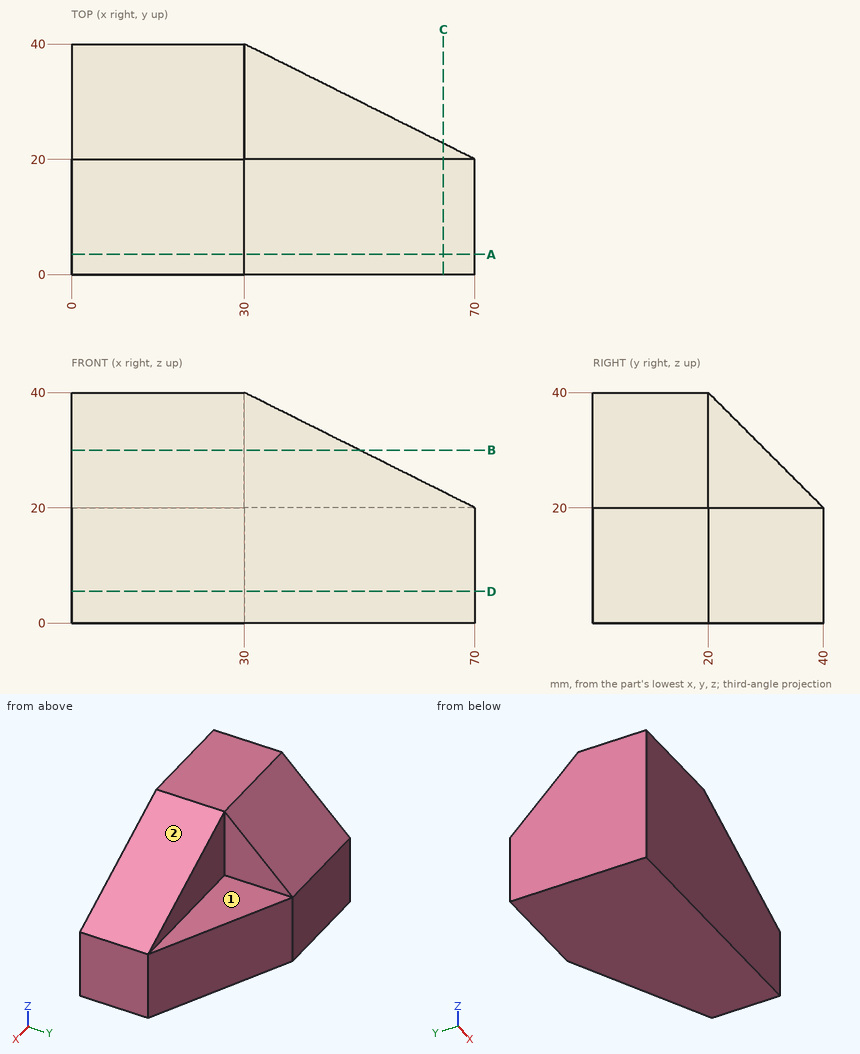
Can you work these out from the drawing? Everything is in mm from the part's minimum corner. A direction names the side the tool comes from. Give positions to 0.01 mm unless a question says otherwise; leave off trailing zeros. Loops run counter-clockwise (first coordinate to the right, second up) from the corner with the lowest first, then second, coordinate; pieces in that order, holes last. Notation, with made-up numbers: (12.5, 55.25) - (39.5, 55.25) arc R30 ccw to (39.5, 89.25) - close; hole circle Ø9 at (62, 10). An arc over 180 degrees is marked (long way). Use one line per item in the form item = value.
1. On a 3-axis mill with a long thin cutter (end or side, diameter ignored), from which of +Z, -Z, +X, -X, +Y, -Y can I reach the whole of each face in a straight line? I mean the marked faces 1 and 2. Say none if no direction works.
Response values:
face_1 = +Z, +X, +Y
face_2 = +Z, +X, +Y, -Y
2. I need wall thicknesses on probe 1 along Z at (x, y) = (38, 24); probe 2 along X at (y, z) = (20.5, 7). Which ranges of each line are inside material? Lowest first, please.
Response values:
probe_1 = 0 to 20
probe_2 = 0 to 69
3. I want a section at B-B (z = 30). Please give me the cut outline in (x, y).
Response values:
outline = (0, 0) - (50, 0) - (50, 20) - (30, 20) - (30, 30) - (0, 30) - close
4. I'm going to push flat-ended pins straight in: pin 1 Ø12 at (y, z) = (31.5, 36) entering from +X; pin 2 Ø6 at (x, z) = (57.5, 16.5) entering from +Y; pin 3 Ø12 at (y, z) = (13.5, 24) entering from -X; pin 4 Ø10 at (x, z) = (45, 29.5) entering from +Y. Where does each tip first touch, or does it pass through?
Response values:
pin_1 = 30
pin_2 = 27.75
pin_3 = 0
pin_4 = 20
5. I want a section at C-C (x = 64.5). Please give me the cut outline in (y, z).
Response values:
outline = (0, 0) - (22.75, 0) - (22.75, 20) - (20, 20) - (20, 22.75) - (0, 22.75) - close
6. I want a section at A-A (y = 3.5). Please give me the cut outline in (x, z).
Response values:
outline = (0, 0) - (70, 0) - (70, 20) - (30, 40) - (0, 40) - close
